Design review of the part built by this model. Coordinates are the model's own, in mm. A direction names the side the tool comes from. Coordinates: 2 decimals unless noted, no trailing zeros. Write each loop counter-clockwise with the first axis right and the second up, starting at its lowest first coordinate (ties: lowest second). Pieces come first, ordered by that corner, then holes.
Q1. Add section B-B, the plane x = -60. Give the boundary of the cut face in (y, z), plus the area to 3 significant figures.
Q2. The part is to be moulded in two halves that separate along Z. For faces 4 (the face through (73, 9, 47)), 5 (the face through (39.17, 12.08, -46.76)), 6 (the face through (-1, 18, -23)), say which applies: +Z half, -Z half, draft (parallel to the pull), parting line (faces both ways), or undercut.
Q3. Add section D-D, the plane x = -11. Give the boundary of the cut face in (y, z).
Q4. Clearance check with flat-ended pins moving along their axes: pin 1 Ø6 at (x, z) = (34, 33.5) entering from +Y; pin 2 Ø4.5 at (x, z) = (-61, 31) entering from -Y; pin 3 Ø12 at (x, z) = (60, -32) entering from -Y. State where each tip first meets the part, or that it passes through.
Q5. Add section A-A, the plane z = 18. Give the boundary of the cut face in (x, y).
Q6. Add section C-C, the plane y = 14.75. Give the number of separate pieces and of enclosed holes in the cut face, plus the area to 3 significant figures.
Q7. Machinability: for faces 1 (the face through (39.17, 12.08, 27.24)), 2 (the face through (-60, 8, -37)), 3 (the face through (-62.08, 13.07, 28.01)), which of the approach directions +Z, -Z, +X, -X, +Y, -Y give a long, thin tool a straight path to every point of the face, cutting with its end or side? Answer none if there is none.
Q8. To check wall thickness, follow probe 1 along Z at (x, y) = (37, 1.5); probe 2 along Z at (x, y) = (60, 13.75); probe 3 along X at (y, z) = (12.5, 43.5). State the ranges of each line that lie inside material, in increasing order.
from build123d import *

# Parameters (mm, degrees)
SKETCH_1_W                    = 150
SKETCH_1_H                    = 100
EXTRUDE_1_DEPTH               = 18
CHAMFER_1_SIZE                = 5
HOLE_WIZARD_M8_1_D            = 9
HOLE_WIZARD_M8_1_CBORE_D      = 15
HOLE_WIZARD_M8_1_CBORE_DEPTH  = 8
HOLE_WIZARD_M12_5_D           = 13.5
HOLE_WIZARD_M12_5_CBORE_D     = 20
HOLE_WIZARD_M12_5_CBORE_DEPTH = 12
SKETCH_16_R                   = 22.5
CUT_EXTRUDE_3_DEPTH           = 92.91844211


with BuildPart() as part:
    # 草圖1 → 伸長1 (new body)
    with BuildSketch(Plane(origin=(0, 0, 0), x_dir=(1, 0, 0), z_dir=(0, 1, 0))):
        Rectangle(SKETCH_1_W, SKETCH_1_H)
    extrude(amount=EXTRUDE_1_DEPTH)

    # 導角1
    chamfer_1_edges = [part.edges().sort_by_distance(p)[0] for p in [
        (-75, 9, -50),
        (75, 9, -50),
        (75, 9, 50),
        (-75, 9, 50),
    ]]
    chamfer(chamfer_1_edges, length=CHAMFER_1_SIZE)

    # M8 六角承窩頭蓋螺釘的柱孔1 (through all)
    with Locations(Plane(origin=(-62.5, 0, 50), x_dir=(1, 0, 0), z_dir=(0, -1, 0))):
        with Locations((2.5, -82), (2.5, -18), (122.5, -18), (122.5, -82)):
            CounterBoreHole(HOLE_WIZARD_M8_1_D / 2, HOLE_WIZARD_M8_1_CBORE_D / 2, HOLE_WIZARD_M8_1_CBORE_DEPTH)

    # M12 六角承窩頭蓋螺釘的柱孔5 (through all)
    with Locations(Plane(origin=(0, 18, 0), x_dir=(-1, 0, 0), z_dir=(0, 1, 0))):
        with Locations((37, -37), (-37, -37), (-37, 37), (37, 37)):
            CounterBoreHole(HOLE_WIZARD_M12_5_D / 2, HOLE_WIZARD_M12_5_CBORE_D / 2, HOLE_WIZARD_M12_5_CBORE_DEPTH)

    # 草圖16 → 除料-伸長3 (cut, through all)
    with BuildSketch(Plane(origin=(0, 18, 0), x_dir=(1, 0, 0), z_dir=(0, 1, 0))):
        with Locations(Location((0, 0, 0), (0, 0, 270))):
            Circle(SKETCH_16_R)
    extrude(amount=-CUT_EXTRUDE_3_DEPTH, mode=Mode.SUBTRACT)


solid = part.part
Here are the results:
1. outline: (0, -50) - (18, -50) - (18, -36.5) - (8, -36.5) - (8, -39.5) - (0, -39.5) - close; (0, -24.5) - (8, -24.5) - (8, -27.5) - (18, -27.5) - (18, 27.5) - (8, 27.5) - (8, 24.5) - (0, 24.5) - close; (0, 39.5) - (8, 39.5) - (8, 36.5) - (18, 36.5) - (18, 50) - (0, 50) - close
1. area: 1,380 mm2
2. face 4: +Z half
2. face 5: undercut
2. face 6: draft
3. outline: (0, -50) - (18, -50) - (18, -19.63) - (0, -19.63) - close; (0, 19.63) - (18, 19.63) - (18, 50) - (0, 50) - close
4. pin 1: stops at y = 6
4. pin 2: passes through
4. pin 3: stops at y = 8
5. outline: (-75, 0) - (-13.5, 0) - (-13.5, 18) - (-75, 18) - close; (13.5, 0) - (75, 0) - (75, 18) - (13.5, 18) - close
6. separate pieces: 1
6. enclosed holes: 9
6. area: 11,800 mm2
7. face 1: +Y
7. face 2: -Y
7. face 3: +Y, -Y
8. probe 1: z = -50 to -43.75, -30.25 to 30.25, 43.75 to 50
8. probe 2: z = -50 to -36.5, -27.5 to 27.5, 36.5 to 50
8. probe 3: x = -75 to -44.6, -29.4 to 29.4, 44.6 to 75
